from build123d import *

# Parameters (mm, degrees)
SKETCH1_R           = 50.8
BOSS_EXTRUDE1_DEPTH = 3.175
SKETCH2_R           = 48.26
CUT_EXTRUDE1_DEPTH  = 0.84582
SKETCH3_R           = 7.9375
CUT_EXTRUDE2_DEPTH  = 21.1328
SKETCH4_R           = 1.7526
CUT_EXTRUDE3_DEPTH  = 72.912172996
SKETCH5_R           = 5.7785
BOSS_EXTRUDE2_DEPTH = 13.5128
FILLET1_R           = 1.27
FILLET2_R           = 1.27


with BuildPart() as part:
    # Sketch1 → Boss-Extrude1 (new body)
    with BuildSketch(Plane.XY):
        Circle(SKETCH1_R)
    extrude(amount=BOSS_EXTRUDE1_DEPTH)

    # Sketch2 → Cut-Extrude1 (cut)
    with BuildSketch(Plane(origin=(0, 0, 0), x_dir=(-1, 0, 0), z_dir=(0, 0, -1))):
        Circle(SKETCH2_R)
    extrude(amount=-CUT_EXTRUDE1_DEPTH, mode=Mode.SUBTRACT)

    # Sketch3 → Cut-Extrude2 (cut)
    with BuildSketch(Plane.XY.offset(3.175)):
        Circle(SKETCH3_R)
    extrude(amount=-CUT_EXTRUDE2_DEPTH, mode=Mode.SUBTRACT)

    # Sketch4 → Cut-Extrude3 (cut, through all)
    with BuildSketch(Plane.XY.offset(3.175)):
        with Locations((27.55148392, 32.834579943)):
            Circle(SKETCH4_R)
        with Locations((-27.55148392, -32.834579943)):
            Circle(SKETCH4_R)
    extrude(amount=-CUT_EXTRUDE3_DEPTH, mode=Mode.SUBTRACT)

    # Sketch5 → Boss-Extrude2 (add)
    with BuildSketch(Plane.XY.offset(3.175)):
        with Locations((-38.1, 0)):
            Circle(SKETCH5_R)
        with Locations((38.1, 0)):
            Circle(SKETCH5_R)
    extrude(amount=BOSS_EXTRUDE2_DEPTH)

    # Sketch8 → 5/32 (0.15625) Diameter Hole1 (revolve, cut)
    with BuildSketch(Plane(origin=(-32.325156325, 0.205530485, 10.329557964), x_dir=(-0.03556813784183403, 0.9993672536012296, 0), z_dir=(0, 0, 1))):
        Polygon((0, 0), (0, 8.761532791), (1.984375, 7.5692), (1.984375, 0), align=None)
    f_5_32_0_15625_diameter_hole1 = revolve(axis=Axis((-25.979174265, 0.43138816, 10.329557964), (-0.9993672536012297, -0.03556813784183403, 0)), mode=Mode.SUBTRACT)

    # Mirror1: 5/32 (0.15625) Diameter Hole1 across plane
    add(f_5_32_0_15625_diameter_hole1.mirror(Plane(origin=(0, 0, 0), x_dir=(0, 0, 1), z_dir=(1, 0, 0))), mode=Mode.SUBTRACT)

    # Fillet1
    fillet1_edges = [part.edges().sort_by_distance(p)[0] for p in [
        (-43.8785, 0, 16.6878),
        (32.3215, 0, 16.6878),
    ]]
    fillet(fillet1_edges, radius=FILLET1_R)

    # Fillet2
    fillet2_edges = [part.edges().sort_by_distance(p)[0] for p in [
        (-50.8, 0, 3.175),
    ]]
    fillet(fillet2_edges, radius=FILLET2_R)


solid = part.part
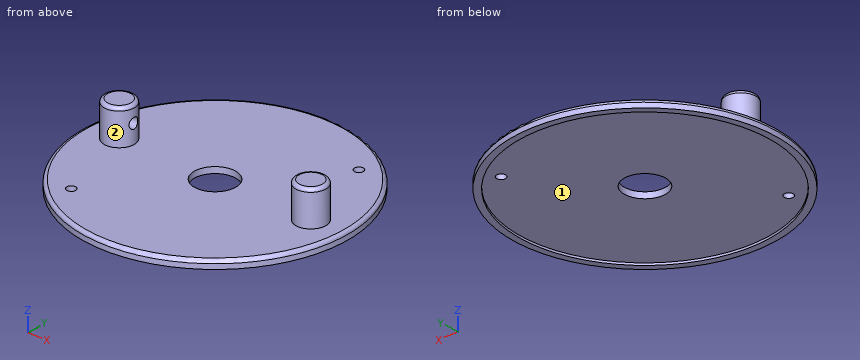
Input: part model. Units: mm. Frame: model coordinates. Face numbers are marked on the shaded views. A direction names the side the tool comes from. Give positions to 0.01 mm unless a question says otherwise; leave off trailing zeros. Order: outer loops, then holes, each group sorted by start corner. A loop starts at its lowest first (then second) coordinate and runs counter-clockwise, first axis right, second up.
Q1. Set-up query: the marked faces 1 and 2. Return all of +Z, -Z, +X, -X, +Y, -Y with unobstructed straight access to the full face (end or side cutting, diameter ignored); none if empty.
Checked values:
face 1: -Z
face 2: +Z
Q2. Section B-B on z = 6. Output: boundary loops of the cut face in (x, y).
Checked values:
outline: circle Ø11.56 at (-38.1, 0); circle Ø11.56 at (38.1, 0)
Q3. Ray query, probe 1 along Y at (x, z) = (0, 0.5); probe 2 along Z at (x, y) = (-42, 10.5) (3 decimals); probe 3 along Y at (x, z) = (-1, 3). Return the intervals inside material, ascending.
Checked values:
probe 1: y = -50.8 to -48.26, 48.26 to 50.8
probe 2: z = 0.846 to 3.175
probe 3: y = -50.16 to -7.87, 7.87 to 50.16
Q4. Section A-A on x = 0. Output: boundary loops of the cut face in (y, z) (1 decimal).
Checked values:
outline: (-50.8, 0) - (-48.3, 0) - (-48.3, 0.8) - (-7.9, 0.8) - (-7.9, 3.2) - (-49.5, 3.2) arc R1.3 ccw to (-50.8, 1.9) - close; (7.9, 0.8) - (48.3, 0.8) - (48.3, 0) - (50.8, 0) - (50.8, 1.9) arc R1.3 ccw to (49.5, 3.2) - (7.9, 3.2) - close
Q5. Contact query for flat-ended pins moving along their axis: pin 1 Ø12.5 at (x, y) = (0, 0) entering from -Z; pin 2 Ø10 at (y, z) = (22.5, 6.5) entering from +X; pin 3 Ø6 at (x, y) = (-28, -29) entering from -Z; pin 4 Ø5.5 at (x, y) = (-27.55, -32.83) entering from +Z (3 decimals). Output: stop coordinate, or through.
Checked values:
pin 1: passes through
pin 2: stops at x = 46.75
pin 3: stops at z = 0.85
pin 4: stops at z = 3.175
